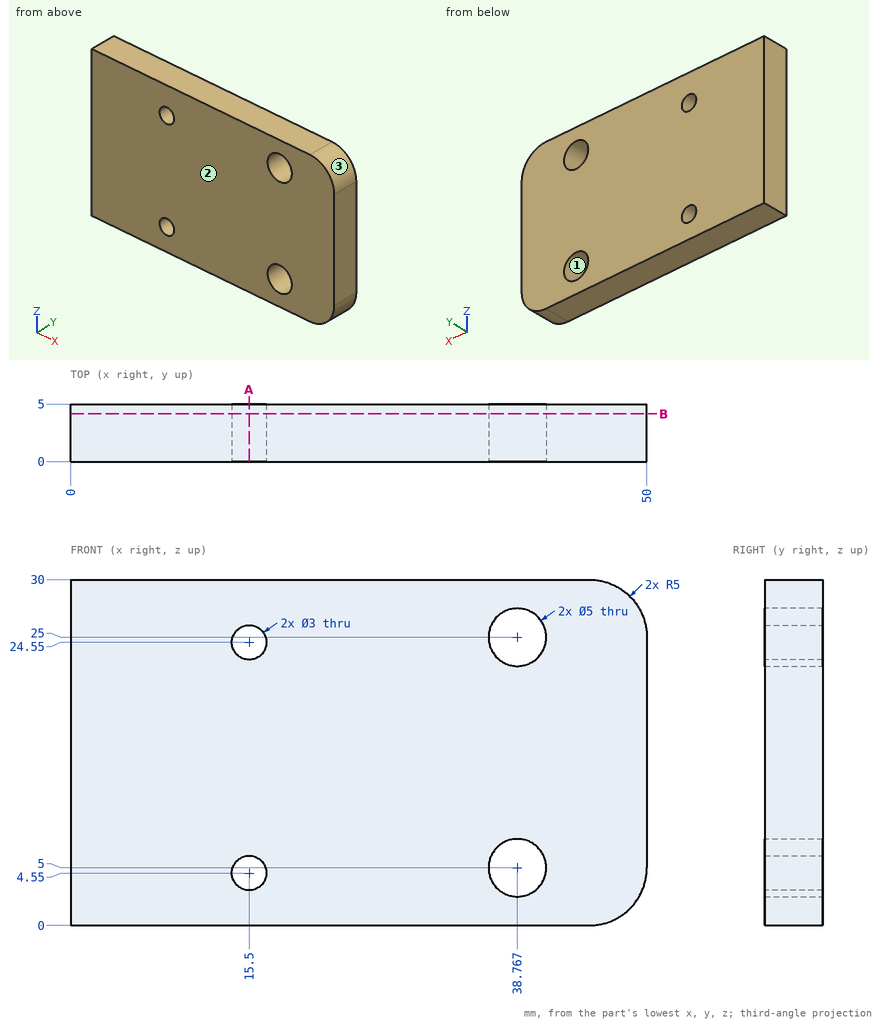
Could you check a few things on this drawing? It's one solid part, dimensions in mm from its lowest x, y, z. Give positions to 0.01 mm unless a question says otherwise; leave off trailing zeros. Order: outer loops, then holes, each group sorted by start corner. A loop starts at its lowest first (then second) coordinate and runs counter-clockwise, first axis right, second up. Notation, with made-up numbers: (10, -6) - (38, -6) arc R20 cw to (38, 1) - close; hole circle Ø1 at (21, 50.25). An arc over 180 degrees is marked (long way). One line per item, written item: value. Start each with the question number.
1. Imagine slicing it at A-A on x = 15.5. List the corners of the cut face in (y, z) for me.
2. If I drill on probe 1 along Z at (x, y) = (37, 3.8); probe 2 along X at (y, z) = (3.5, 25); probe 3 along X at (y, z) = (1.55, 4.55), over which ranges is the centre line in solid material (lowest first)?
3. Imagine slicing it at B-B on y = 4.15. List the corners of the cut face in (x, z) for me, plus the area to 3 significant figures.
4. Thinking about a two-plate mould opening in Z: for the marked faces 1, 2 and 3, which applies, +Z half, -Z half, draft (parallel to the pull), parting line (faces both ways), or undercut?
5. For P1, Ø4, axis at x = 38.77, z = 25, coming from the +Y side, with a flat end and sliding along its axis, tell me the tip position at first contact or that it passes through.
Values:
1. outline: (0, 0) - (5, 0) - (5, 3.05) - (0, 3.05) - close; (0, 6.05) - (5, 6.05) - (5, 23.05) - (0, 23.05) - close; (0, 26.05) - (5, 26.05) - (5, 30) - (0, 30) - close
2. probe 1: 0 to 3.23, 6.77 to 23.23, 26.77 to 30
2. probe 2: 0 to 14.07, 16.93 to 36.27, 41.27 to 50
2. probe 3: 0 to 14, 17 to 36.31, 41.23 to 49.98
3. outline: (0, 0) - (45, 0) arc R5 ccw to (50, 5) - (50, 25) arc R5 ccw to (45, 30) - (0, 30) - close; hole circle Ø3 at (15.5, 4.55); hole circle Ø3 at (15.5, 24.55); hole circle Ø5 at (38.77, 5); hole circle Ø5 at (38.77, 25)
3. area: 1,440 mm²
4. face 1: undercut
4. face 2: draft
4. face 3: +Z half
5. P1: through
